from build123d import *

# Parameters (mm, degrees)
EXTRUDE_1_DEPTH     = 5
SKETCH_3_R          = 1.5
CUT_EXTRUDE_1_DEPTH = 9
SKETCH_4_R          = 3
CUT_EXTRUDE_2_DEPTH = 5


with BuildPart() as part:
    # 草圖1 → 填料-伸長1 (new body, symmetric)
    with BuildSketch(Plane.XY):
        with BuildLine():
            Line((-4.116062299, 0), (4.116062299, 0))
            ThreePointArc((4.116062299, 0), (6.42113368, -2.146292611), (7.753905297, -5))
            Line((7.753905297, -5), (11, -5))
            Line((11, -5), (11, -8))
            Line((11, -8), (6, -8))
            Line((6, -8), (6, -7))
            ThreePointArc((6, -7), (5.340169944, -4.204915028), (3.5, -2))
            Line((3.5, -2), (-3.5, -2))
            ThreePointArc((-3.5, -2), (-5.340169944, -4.204915028), (-6, -7))
            Line((-6, -7), (-6, -8))
            Line((-6, -8), (-11, -8))
            Line((-11, -8), (-11, -5))
            Line((-11, -5), (-7.753905297, -5))
            ThreePointArc((-7.753905297, -5), (-6.42113368, -2.146292611), (-4.116062299, 0))
        make_face()
    extrude(amount=EXTRUDE_1_DEPTH, both=True)

    # 草圖3 → 除料-伸長1 (cut, through all)
    with BuildSketch(Plane.XZ.offset(8)):
        with Locations((-8.5, 0)):
            Circle(SKETCH_3_R)
        with Locations((8.5, 0)):
            Circle(SKETCH_3_R)
    extrude(amount=-CUT_EXTRUDE_1_DEPTH, mode=Mode.SUBTRACT)

    # 草圖4 → 除料-伸長2 (cut)
    with BuildSketch(Plane(origin=(0, 0, 0), x_dir=(1, 0, 0), z_dir=(0, 1, 0))):
        with Locations((8.5, 0)):
            Circle(SKETCH_4_R)
        with Locations((-8.5, 0)):
            Circle(SKETCH_4_R)
    extrude(amount=-CUT_EXTRUDE_2_DEPTH, mode=Mode.SUBTRACT)


solid = part.part
Source: CAD feature listing. Evaluate the final solid. Frame: model axes, mm. A direction names the side the tool comes from. Round coordinates to 2 decimals unless told otherwise and drop trailing zeros. Loops run counter-clockwise (first coordinate to the right, second up) from the corner with the lowest first, then second, coordinate; pieces in that order, holes last.
Q1. Access query for faces 1 (the face through (5.5, -3.4, -0.1)), 2 (the face through (5.468, -1.053, -1.041)), 3 (the face through (0.9, -1.6, -5)), 4 (the face through (-6, -7.5, 0.1)), 5 (the face through (-10, -5, 1)). Directions: +Z, -Z, +X, -X, +Y, -Y. A direction counts if a zero-diameter tool reaches every point of the face in a straight line with its end or side. Return the directions, or none.
Q2. Mould query, pull axis X, two halves, no side actions, for faces 6 (the face through (10, -5, -1)), 7 (the face through (-10, -7, 0)), 8 (the face through (11, -6, 0)), 9 (the face through (0, -2, 0)). Classes: pulls with the +X half, pulls with the -X half, needs draft (parallel to the pull), parting line crosses it, or undercut.
Q3. First-contact query: P1, Ø4.5, axis at x = 8, z = 1, coming from the +Y side; P2, Ø5.5, axis at x = -0.5, z = -2.5, coming from the -Y side; P3, Ø1.8, axis at x = 8.5, z = 0, coming from the -Y side. Flat tips, straight axial feed; report the tip coordinate or a pass-through.
Q4. Section A-A, the plane y = -7.25. Return loops of the section in (x, z).
Q5. Section C-C, the plane y = -3.5. Return loops of the section in (x, z), plus the area to 3 significant figures.
Q6. Section D-D, the plane z = -1.25. Return loops of the section in (x, y), plus the area to 3 significant figures.
Q7. Ray query, line 1 (X direction, y = -6.75, z = -2.5) (3 decimals); line 2 (Z direction, x = -8.5, y = -6.9); line 3 (Y direction, x = -0.75, z = -1.5). Return the intervals inside material, ascending.
Q8. Section B-B, the plane x = -8.5. Return loops of the section in (y, z).
Solutions:
1. face 1: +X, +Y
1. face 2: +Z, -Z, +X, +Y
1. face 3: -Z, +X, -X, +Y, -Y
1. face 4: +Z, -Z, -Y
1. face 5: -X, +Y
2. face 6: needs draft
2. face 7: undercut
2. face 8: pulls with the +X half
2. face 9: undercut
3. P1: stops at y = -1.35
3. P2: stops at y = -2
3. P3: passes through
4. outline: (-11, -5) - (-6, -5) - (-6, 5) - (-11, 5) - close; (6, -5) - (11, -5) - (11, 5) - (6, 5) - close; hole circle Ø3 at (-8.5, 0); hole circle Ø3 at (8.5, 0)
5. outline: (-7.22, -5) - (-4.93, -5) - (-4.93, 5) - (-7.22, 5) - (-7.22, 2.71) arc R3 cw to (-7.22, -2.71) - close; (4.93, -5) - (7.22, -5) - (7.22, -2.71) arc R3 cw to (7.22, 2.71) - (7.22, 5) - (4.93, 5) - close
5. area: 32.5 mm2
6. outline: (-11, -8) - (-9.33, -8) - (-9.33, -5) - (-11, -5) - close; (-7.67, -8) - (-6, -8) - (-6, -7) arc R6.25 cw to (-3.5, -2) - (3.5, -2) arc R6.25 cw to (6, -7) - (6, -8) - (7.67, -8) - (7.67, -5) - (5.77, -5) - (5.77, -1.36) arc R8.25 ccw to (4.12, 0) - (-4.12, 0) arc R8.25 ccw to (-5.77, -1.36) - (-5.77, -5) - (-7.67, -5) - close; (9.33, -8) - (11, -8) - (11, -5) - (9.33, -5) - close
6. area: 47.2 mm2
7. line 1: x = -11 to -5.995, 5.995 to 11
7. line 2: z = -5 to -1.5, 1.5 to 5
7. line 3: y = -2 to 0
8. outline: (-8, -5) - (-5, -5) - (-5, -1.5) - (-8, -1.5) - close; (-8, 1.5) - (-5, 1.5) - (-5, 5) - (-8, 5) - close
